from build123d import *

# Parameters (mm, degrees)
F0_W      = 23.5
F0_H      = 23.5
F1_DEPTH  = 11.75
F2_W      = 20
F2_H      = 20
F3_DEPTH  = 47
F4_SIZE   = 2
F5_R      = 3.75
F6_DEPTH  = 47
F7_SIZE2  = 4
F7_SIZE   = 2
F8_W      = 20
F8_H      = 20
F9_DEPTH  = 48
F10_R     = 3.3166247904
F11_DEPTH = 48
F12_SIZE  = 2
F13_SIZE2 = 5
F13_SIZE  = 2
F14_DEPTH = 48
F15_DEPTH = 48


with BuildPart() as f1:
    # F0 (on Top) → F1 (new body, symmetric)
    with BuildSketch(Plane.XY):
        Rectangle(F0_W, F0_H)
    extrude(amount=F1_DEPTH, both=True)

    # F2 (on face) → F3 (join)
    with BuildSketch(Plane.YZ.offset(11.75)):
        Rectangle(F2_W, F2_H)
    extrude(amount=F3_DEPTH)

    # F4
    f4_edges = [f1.edges().sort_by_distance(p)[0] for p in [
        (35.25, -10, 10),
        (35.25, -10, -10),
        (35.25, 10, 10),
        (35.25, 10, -10),
    ]]
    chamfer(f4_edges, length=F4_SIZE)

    # F5 (on face) → F6 (cut, through all)
    with BuildSketch(Plane.YZ.offset(58.75)):
        with Locations((0, 11.75)):
            Circle(F5_R)
        with Locations((11.75, 0)):
            Circle(F5_R)
        with Locations((0, -11.75)):
            Circle(F5_R)
        with Locations((-11.75, 0)):
            Circle(F5_R)
    extrude(amount=-F6_DEPTH, mode=Mode.SUBTRACT)

    # F7
    f7_edges = [f1.edges().sort_by_distance(p)[0] for p in [
        (58.75, -9, -9),
        (58.75, -5.658312, -10),
        (58.75, 0, -8),
        (58.75, 5.658312, -10),
        (58.75, 9, -9),
        (58.75, 10, -5.658312),
        (58.75, 8, 0),
        (58.75, 10, 5.658312),
        (58.75, 9, 9),
        (58.75, 5.658312, 10),
        (58.75, 0, 8),
        (58.75, -5.658312, 10),
        (58.75, -9, 9),
        (58.75, -10, 5.658312),
        (58.75, -8, 0),
        (58.75, -10, -5.658312),
    ]]
    f7_side = f1.faces().sort_by_distance((58.75, 0, 0))[0]
    chamfer(f7_edges, length=F7_SIZE, length2=F7_SIZE2, reference=f7_side)

    # F8 (on face) → F9 (join)
    with BuildSketch(Plane.XZ.offset(11.75)):
        Rectangle(F8_W, F8_H)
    extrude(amount=F9_DEPTH)

    # F10 (on face) → F11 (cut)
    with BuildSketch(Plane.XZ.offset(59.75)):
        with Locations((11.3166247904, 0)):
            Circle(F10_R)
        with Locations((0, 11.3166247904)):
            Circle(F10_R)
        with Locations((-11.3166247904, 0)):
            Circle(F10_R)
        with Locations((0, -11.3166247904)):
            Circle(F10_R)
    extrude(amount=-F11_DEPTH, mode=Mode.SUBTRACT)

    # F12
    f12_edges = [f1.edges().sort_by_distance(p)[0] for p in [
        (10, -35.75, 10),
        (10, -35.75, -10),
        (-10, -35.75, 10),
        (-10, -35.75, -10),
    ]]
    chamfer(f12_edges, length=F12_SIZE)

    # F13
    f13_edges = [f1.edges().sort_by_distance(p)[0] for p in [
        (-10, -59.75, -5.522046),
        (-9, -59.75, -9),
        (-8, -59.75, 0),
        (-5.522046, -59.75, -10),
        (-10, -59.75, 5.522046),
        (0, -59.75, -8),
        (-9, -59.75, 9),
        (5.522046, -59.75, -10),
        (-5.522046, -59.75, 10),
        (9, -59.75, -9),
        (0, -59.75, 8),
        (10, -59.75, -5.522046),
        (5.522046, -59.75, 10),
        (8, -59.75, 0),
        (9, -59.75, 9),
        (10, -59.75, 5.522046),
    ]]
    f13_side = f1.faces().sort_by_distance((0, -59.75, 0))[0]
    chamfer(f13_edges, length=F13_SIZE, length2=F13_SIZE2, reference=f13_side)

    # F14 (cut): a face of the model
    f14_faces = [f1.faces().sort_by_distance(p)[0] for p in [
        (58.75, 0, 0),
    ]]
    extrude(f14_faces, amount=-F14_DEPTH, mode=Mode.SUBTRACT)

    # F15 (cut): a face of the model
    f15_faces = [f1.faces().sort_by_distance(p)[0] for p in [
        (0, -59.75, 0),
    ]]
    extrude(f15_faces, amount=-F15_DEPTH, mode=Mode.SUBTRACT)


solid = f1.part
Source: CAD feature listing. Evaluate the final solid. Frame: model axes, mm. A direction names the side the tool comes from. Coordinates: 2 decimals unless noted, no trailing zeros.
Item 1: First-contact query: P1, Ø1.5, axis at x = 42.5, y = -4.5, coming from the -Z side; P2, Ø1.5, axis at y = -26, z = -5.5, coming from the -X side; P3, Ø3, axis at x = 28.5, y = 6.5, coming from the +Z side. Flat tips, straight axial feed; report the tip coordinate or a pass-through.
Output values:
P1: stops at z = -10
P2: stops at x = -10
P3: stops at z = 10
Item 2: Pull-direction query (Z, two-part tool) for faces 5 (the face through (34, -8, 0)), 6 (the face through (0, -34, 8)), 7 (the face through (33, 6, -10)); classes: pulls with the +Z half, pulls with the -Z half, needs draft (parallel to the pull), parting line crosses it, or undercut.
Output values:
face 5: undercut
face 6: pulls with the +Z half
face 7: pulls with the -Z half
Item 3: Set-up query: faces 1 (the face through (-6, -33, -10)), 2 (the face through (33, -9, -9)), 3 (the face through (34, 0, 8)), 4 (the face through (35, -6, 0)). Return all of +Z, -Z, +X, -X, +Y, -Y with unobstructed straight access to the full face (end or side cutting, diameter ignored); none if empty.
Output values:
face 1: -Z, +X, -X, -Y
face 2: -Z, +X, -Y
face 3: +Z, +X
face 4: +X
Item 4: Material intervals for line 1 (X direction, y = -39.5, z = 7.5); line 2 (Y direction, x = 36, z = -7); line 3 (X direction, y = -29, z = -5.75), sorted ascending.
Output values:
line 1: x = -10 to -7.67, -3.7 to 3.7, 7.67 to 10
line 2: y = -10 to -8, -3.24 to 3.24, 8 to 10
line 3: x = -10 to -8, 8 to 10
